```python
from build123d import *

# Parameters (mm, degrees)
F1_DEPTH = 150
F2_R     = 5


with BuildPart() as f1:
    # F0 (on Front) → F1 (new body)
    with BuildSketch(Plane.XZ):
        with BuildLine():
            ThreePointArc((0, 35), (1.464466, 38.535534), (5, 40))
            Line((5, 40), (35, 40))
            ThreePointArc((35, 40), (38.535534, 38.535534), (40, 35))
            Line((40, 35), (40, 5))
            ThreePointArc((40, 5), (41.464466, 1.464466), (45, 0))
            Line((45, 0), (75, 0))
            ThreePointArc((75, 0), (78.535534, 1.464466), (80, 5))
            Line((80, 5), (80, 35))
            ThreePointArc((80, 35), (81.464466, 38.535534), (85, 40))
            Line((85, 40), (115, 40))
            ThreePointArc((115, 40), (118.535534, 38.535534), (120, 35))
            Line((120, 35), (120, 5))
            ThreePointArc((120, 5), (121.464466, 1.464466), (125, 0))
            Line((125, 0), (160, 0))
            Line((160, 0), (160, 2))
            Line((160, 2), (122, 2))
            Line((122, 2), (122, 35))
            ThreePointArc((122, 35), (119.949747, 39.949747), (115, 42))
            Line((115, 42), (85, 42))
            ThreePointArc((85, 42), (80.050253, 39.949747), (78, 35))
            Line((78, 35), (78, 2))
            Line((78, 2), (42, 2))
            Line((42, 2), (42, 35))
            ThreePointArc((42, 35), (39.949747, 39.949747), (35, 42))
            Line((35, 42), (5, 42))
            ThreePointArc((5, 42), (0.050253, 39.949747), (-2, 35))
            Line((-2, 35), (-2, 0))
            Line((-2, 0), (0, 0))
            Line((0, 0), (0, 35))
        make_face()
    extrude(amount=F1_DEPTH)

    # F2
    f2_edges = [f1.edges().sort_by_distance(p)[0] for p in [
        (42, -75, 2),
        (122, -75, 2),
    ]]
    fillet(f2_edges, radius=F2_R)


solid = f1.part
```
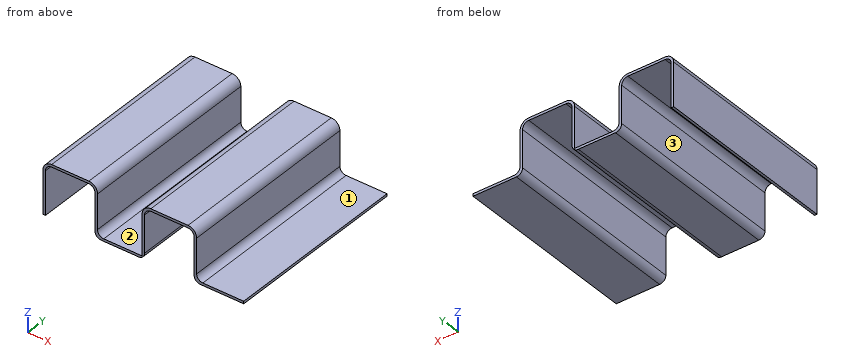
Design review of the part built by this model. Coordinates are the model's own, in mm. Face numbers are marked on the shaded views. A direction names the side the tool comes from. Give positions to 0.01 mm unless a question says otherwise; leave off trailing zeros. Write each loop counter-clockwise with the first axis right and the second up, starting at its lowest first coordinate (ties: lowest second). Pieces come first, ordered by that corner, then holes. Notation, with made-up numbers: (44.5, -9.75) - (72.5, -9.75) arc R18 ccw to (72.5, 24.25) - close; hole circle Ø1 at (83, 82.5). An arc over 180 degrees is marked (long way). Return JSON: item names as keys, results as strings. Group by question number.
(1) To check wall thickness, follow probe 1 along X at (y, z) = (-19.5, 14); probe 2 along X at (y, z) = (-87, 38); probe 3 along Z at (x, y) = (141, -100.5). State the ranges of each line that lie inside material, in increasing order.
(2) Insertion check: pin 1 (2 mm diameter, centred on x = 57.5, y = -131, fed in from +Z); pin 2 (12 mm diameter, centred on x = 70, z = 16.5, fed in from +Y); pin 3 (8 mm diameter, centred on y = -17.5, z = 16, fed in from +X); pin 4 (24 mm diameter, centred on x = 97.5, y = -85.5, fed in from -Z). Each pin has a flat end and moves straight along its axis. Give the tip position at first contact, or say it passes through.
(3) We need section C-C, the plane x = 87. Give the boundary of the cut face in (y, z).
(4) We need section D-D, the plane x = 117.5. Give the boundary of the cut face in (y, z), then the cut area to 3 significant figures.
(5) Machinability: for the marked faces 1, 2 and 3, which of the approach directions +Z, -Z, +X, -X, +Y, -Y give a long, thin tool a straight path to every point of the face, cutting with its end or side? Answer none if there is none.
(6) We need section A-A, the plane z = 26.5. Give the boundary of the cut face in (x, y), then the cut area to 3 significant figures.
Reported:
{
 "1": {"probe 1": "x = -2 to 0, 40 to 42, 78 to 80, 120 to 122", "probe 2": "x = -1.32 to 1, 39 to 41.32, 78.68 to 81, 119 to 121.32", "probe 3": "z = 0 to 2"},
 "2": {"pin 1": "stops at z = 2", "pin 2": "passes through", "pin 3": "stops at x = 122", "pin 4": "stops at z = 40"},
 "3": {"outline": "(-150, 40) - (0, 40) - (0, 42) - (-150, 42) - close"},
 "4": {"outline": "(-150, 39.33) - (0, 39.33) - (0, 41.54) - (-150, 41.54) - close", "area": "331 mm2"},
 "5": {"face 1": "+Z, +X, +Y, -Y", "face 2": "+Z, +Y, -Y", "face 3": "-Z, +Y, -Y"},
 "6": {"outline": "(-2, -150) - (0, -150) - (0, 0) - (-2, 0) - close; (40, -150) - (42, -150) - (42, 0) - (40, 0) - close; (78, -150) - (80, -150) - (80, 0) - (78, 0) - close; (120, -150) - (122, -150) - (122, 0) - (120, 0) - close", "area": "1,200 mm2"}
}
